Source: CAD feature listing. Evaluate the final solid. Frame: model axes, mm. A direction names the side the tool comes from. Round coordinates to 2 decimals unless told otherwise and drop trailing zeros. Loops run counter-clockwise (first coordinate to the right, second up) from the corner with the lowest first, then second, coordinate; pieces in that order, holes last.
(1) First-contact query: pin 1 Ø7 at (x, y) = (-6.5, 19.5) entering from +Z; pin 2 Ø3 at (x, y) = (-34, 20.5) entering from +Z; pin 3 Ø4 at (x, z) = (-15.5, 6) entering from +Y. Flat tips, straight axial feed; report the tip coordinate or a pass-through.
(2) Section C-C, the plane z = 1. Return the cut outline in (x, y), plus the area to 3 significant figures.
(3) Material intervals for probe 1 along X at (y, z) = (20, 2.9); probe 2 along X at (y, z) = (5.75, 5.5); probe 3 along X at (y, z) = (24.5, 2), sorted ascending.
(4) Section D-D, the plane z = 6. Return the cut outline in (x, y).
(5) Section B-B, the plane x = -15.05. Return the cut outline in (y, z), plus the area to 3 significant figures.
(6) Set-up query: faces 1 (the cylindrical face through (-5.98, 16.9, 6.35)), 2 (the flat face through (-30, 18, 4)), 3 (the flat face through (-19.7, 8.1, 11.3)). Return all of +Z, -Z, +X, -X, +Y, -Y with unobstructed straight access to the full face (end or side cutting, diameter ignored); none if empty.
(7) Section A-A, the plane y = 15. Return the cut outline in (x, z), plus the area to 3 significant figures.
(8) Mould query, pull axis Z, two halves, no side actions, for faces 4 (the cylindrical face through (-13.586, 5.07, 5.825)), 5 (the flat face through (-20, 10, 5)), 6 (the flat face through (-34.3, 21.5, 5)). Classes: pulls with the +Z half, pulls with the -Z half, needs draft (parallel to the pull), parting line crosses it, or undercut.
```python
from build123d import *

# Parameters (mm, degrees)
EXTRUDE1_DEPTH = 40
SKETCH2_W      = 20
SKETCH2_H      = 20
EXTRUDE2_DEPTH = 52.923019943
SKETCH3_R      = 1.5
EXTRUDE3_DEPTH = 52.923019943
SKETCH4_R      = 1.5
EXTRUDE4_DEPTH = 47.861498055
SKETCH8_R      = 3.25
EXTRUDE5_DEPTH = 9


with BuildPart() as part:
    # Sketch1 → Extrude1 (new body)
    with BuildSketch(Plane(origin=(0, 0, 0), x_dir=(0, 0, -1), z_dir=(1, 0, 0))):
        Polygon((0, 0), (-14, 0), (-4, 30), (0, 30), align=None)
    extrude(amount=-EXTRUDE1_DEPTH)

    # Sketch2 → Extrude2 (cut, through all)
    with BuildSketch(Plane(origin=(0, 0, 0), x_dir=(-1, 0, 0), z_dir=(0, 0, -1))):
        with Locations((20, 20)):
            Rectangle(SKETCH2_W, SKETCH2_H)
    extrude(amount=-EXTRUDE2_DEPTH, mode=Mode.SUBTRACT)

    # Sketch3 → Extrude3 (cut, through all)
    with BuildSketch(Plane(origin=(0, 0, 0), x_dir=(-1, 0, 0), z_dir=(0, 0, -1))):
        with Locations(Location((5, 20, 0), (0, 0, 90))):
            Circle(SKETCH3_R)
        with Locations(Location((35, 20, 0), (0, 0, 90))):
            Circle(SKETCH3_R)
    extrude(amount=-EXTRUDE3_DEPTH, mode=Mode.SUBTRACT)

    # Sketch4 → Extrude4 (cut, through all)
    with BuildSketch(Plane(origin=(0, 10, 0), x_dir=(1, 0, 0), z_dir=(0, 1, 0))):
        with Locations(Location((-24.95, -5.5, 0), (0, 0, 270))):
            Circle(SKETCH4_R)
        with Locations(Location((-15.05, -5.5, 0), (0, 0, 90))):
            Circle(SKETCH4_R)
    extrude(amount=-EXTRUDE4_DEPTH, mode=Mode.SUBTRACT)

    # Sketch8 → Extrude5 (cut)
    with BuildSketch(Plane(origin=(0, 0, 14), x_dir=(-1, 0, 0), z_dir=(0, 0, -1))):
        with Locations(Location((5, 20, 0), (0, 0, 270))):
            Circle(SKETCH8_R)
        with Locations(Location((35, 20, 0), (0, 0, 270))):
            Circle(SKETCH8_R)
    extrude(amount=EXTRUDE5_DEPTH, mode=Mode.SUBTRACT)


solid = part.part
```
Output values:
1. pin 1: stops at z = 8.67
1. pin 2: stops at z = 5
1. pin 3: stops at y = 10
2. outline: (-40, 0) - (0, 0) - (0, 30) - (-10, 30) - (-10, 10) - (-30, 10) - (-30, 30) - (-40, 30) - close; hole circle Ø3 at (-35, 20); hole circle Ø3 at (-5, 20)
2. area: 786 mm2
3. probe 1: x = -40 to -36.5, -33.5 to -30, -10 to -6.5, -3.5 to 0
3. probe 2: x = -40 to -26.45, -23.45 to -16.55, -13.55 to 0
3. probe 3: x = -40 to -30, -10 to 0
4. outline: (-40, 0) - (-26.36, 0) - (-26.36, 10) - (-30, 10) - (-30, 24) - (-40, 24) - close; (-23.54, 0) - (-16.46, 0) - (-16.46, 10) - (-23.54, 10) - close; (-13.64, 0) - (0, 0) - (0, 24) - (-10, 24) - (-10, 10) - (-13.64, 10) - close; hole circle Ø6.5 at (-35, 20); hole circle Ø6.5 at (-5, 20)
5. outline: (0, 0) - (10, 0) - (10, 4) - (0, 4) - close; (0, 7) - (10, 7) - (10, 10.67) - (0, 14) - close
5. area: 93.3 mm2
6. face 1: +Z
6. face 2: +Z, -Z, +Y
6. face 3: +Z, +X, -X, +Y
7. outline: (-40, 0) - (-30, 0) - (-30, 9) - (-40, 9) - close; (-10, 0) - (0, 0) - (0, 9) - (-10, 9) - close
7. area: 180 mm2
8. face 4: undercut
8. face 5: needs draft
8. face 6: pulls with the +Z half
